```python
from build123d import *

# Parameters (mm, degrees)
SCHIZZO1_R                   = 1.5
ESTRUSIONE_ESTRUSIONE1_DEPTH = 2
TAGLIO_ESTRUSIONE1_DEPTH     = 2
ESTRUSIONE_ESTRUSIONE2_DEPTH = 2


with BuildPart() as part:
    # Schizzo1 → Estrusione-Estrusione1 (new body)
    with BuildSketch(Plane.XY):
        with BuildLine():
            Line((4.009057919, 37.078949925), (4.009057919, -12.921050075))
            ThreePointArc((4.009057919, -12.921050075), (2.544591824, -16.456583981), (-0.990942081, -17.921050075))
            Line((-0.990942081, -17.921050075), (-50.990942081, -17.921050075))
            ThreePointArc((-50.990942081, -17.921050075), (-54.526475987, -16.456583981), (-55.990942081, -12.921050075))
            Line((-55.990942081, -12.921050075), (-55.990942081, 37.078949925))
            ThreePointArc((-55.990942081, 37.078949925), (-54.526475987, 40.614483831), (-50.990942081, 42.078949925))
            Line((-50.990942081, 42.078949925), (-0.990942081, 42.078949925))
            ThreePointArc((-0.990942081, 42.078949925), (2.544591824, 40.614483831), (4.009057919, 37.078949925))
        make_face()
        with Locations((-50.990942081, 37.078949925)):
            Circle(SCHIZZO1_R, mode=Mode.SUBTRACT)
        with Locations((-0.990942081, 37.078949925)):
            Circle(SCHIZZO1_R, mode=Mode.SUBTRACT)
        with Locations((-50.990942081, -12.921050075)):
            Circle(SCHIZZO1_R, mode=Mode.SUBTRACT)
        with Locations((-0.990942081, -12.921050075)):
            Circle(SCHIZZO1_R, mode=Mode.SUBTRACT)
        with BuildLine():
            Line((-31.315733716, 32.226325066), (-29.922818488, 39.296413949))
            ThreePointArc((-29.922818488, 39.296413949), (-36.65420027, 37.427419796), (-42.697428035, 33.922560594))
            Line((-42.697428035, 33.922560594), (-36.878383255, 29.847848476))
            ThreePointArc((-36.878383255, 29.847848476), (-34.183829904, 31.240022968), (-31.315733716, 32.226325066))
        make_face(mode=Mode.SUBTRACT)
        with BuildLine():
            Line((-22.358446359, 39.337984663), (-21.125016906, 32.342042069))
            ThreePointArc((-21.125016906, 32.342042069), (-18.235263935, 31.421121146), (-15.509792769, 30.090491783))
            Line((-15.509792769, 30.090491783), (-9.525545173, 34.104859773))
            ThreePointArc((-9.525545173, 34.104859773), (-15.606929318, 37.543087038), (-22.358446359, 39.337984663))
        make_face(mode=Mode.SUBTRACT)
        with BuildLine():
            Line((-4.147331412, 28.785435879), (-8.22204353, 22.966391099))
            ThreePointArc((-8.22204353, 22.966391099), (-6.829869038, 20.271837748), (-5.84356694, 17.403741559))
            Line((-5.84356694, 17.403741559), (1.226521943, 16.010826332))
            ThreePointArc((1.226521943, 16.010826332), (-0.642472211, 22.742208114), (-4.147331412, 28.785435879))
        make_face(mode=Mode.SUBTRACT)
        with BuildLine():
            Line((1.268092656, 8.446454203), (-5.727849938, 7.213024749))
            ThreePointArc((-5.727849938, 7.213024749), (-6.648770861, 4.323271778), (-7.979400223, 1.597800612))
            Line((-7.979400223, 1.597800612), (-3.965032233, -4.386446983))
            ThreePointArc((-3.965032233, -4.386446983), (-0.526804968, 1.694937161), (1.268092656, 8.446454203))
        make_face(mode=Mode.SUBTRACT)
        with BuildLine():
            Line((-9.284456128, -9.764660744), (-15.103500908, -5.689948626))
            ThreePointArc((-15.103500908, -5.689948626), (-16.317583854, -6.379009649), (-17.575076336, -6.985239929))
            Line((-17.575076336, -6.985239929), (-22.566296054, 5.239602614))
            ThreePointArc((-22.566296054, 5.239602614), (-26.23827157, 19.723797875), (-28.966350145, 5.032545245))
            Line((-28.966350145, 5.032545245), (-34.305917557, -7.029459582))
            ThreePointArc((-34.305917557, -7.029459582), (-35.404993092, -6.512601237), (-36.472091394, -5.932591934))
            Line((-36.472091394, -5.932591934), (-42.45633899, -9.946959923))
            ThreePointArc((-42.45633899, -9.946959923), (-25.839815546, -15.420634813), (-9.284456128, -9.764660744))
        make_face(mode=Mode.SUBTRACT)
        with BuildLine():
            Line((-47.834552751, -4.627536029), (-43.759840633, 1.191508751))
            ThreePointArc((-43.759840633, 1.191508751), (-45.152015125, 3.886062102), (-46.138317223, 6.754158291))
            Line((-46.138317223, 6.754158291), (-53.208406106, 8.147073518))
            ThreePointArc((-53.208406106, 8.147073518), (-51.339411952, 1.415691736), (-47.834552751, -4.627536029))
        make_face(mode=Mode.SUBTRACT)
        with BuildLine():
            Line((-53.249976819, 15.711445647), (-46.254034225, 16.944875101))
            ThreePointArc((-46.254034225, 16.944875101), (-45.333113302, 19.834628071), (-44.00248394, 22.560099238))
            Line((-44.00248394, 22.560099238), (-48.01685193, 28.544346833))
            ThreePointArc((-48.01685193, 28.544346833), (-51.455079195, 22.462962688), (-53.249976819, 15.711445647))
        make_face(mode=Mode.SUBTRACT)
    extrude(amount=ESTRUSIONE_ESTRUSIONE1_DEPTH)

    # Schizzo2 → Taglio-Estrusione1 (cut)
    with BuildSketch(Plane.XY):
        with BuildLine():
            Line((-29.267736933, 24.477334627), (-28.432897549, 28.714770282))
            Line((-28.432897549, 28.714770282), (-23.731058754, 28.714770282))
            Line((-23.731058754, 28.714770282), (-22.996526589, 24.54854509))
            ThreePointArc((-22.996526589, 24.54854509), (-21.218217068, 23.981824522), (-19.541004043, 23.162975684))
            Line((-19.541004043, 23.162975684), (-15.954363967, 25.56897458))
            Line((-15.954363967, 25.56897458), (-12.629661871, 22.244272484))
            Line((-12.629661871, 22.244272484), (-15.056235281, 18.778913724))
            ThreePointArc((-15.056235281, 18.778913724), (-14.199512517, 17.120727047), (-13.592557379, 15.355744777))
            Line((-13.592557379, 15.355744777), (-9.355121725, 14.520905393))
            Line((-9.355121725, 14.520905393), (-9.355121725, 9.819066597))
            Line((-9.355121725, 9.819066597), (-13.521346916, 9.084534432))
            ThreePointArc((-13.521346916, 9.084534432), (-14.088067484, 7.306224912), (-14.906916322, 5.629011886))
            Line((-14.906916322, 5.629011886), (-12.500917426, 2.042371811))
            Line((-12.500917426, 2.042371811), (-15.825619522, -1.282330286))
            Line((-15.825619522, -1.282330286), (-19.290978282, 1.144243124))
            ThreePointArc((-19.290978282, 1.144243124), (-20.038106249, 0.720205572), (-20.811947777, 0.347140784))
            Line((-20.811947777, 0.347140784), (-23.883467603, 7.870120811))
            ThreePointArc((-23.883467603, 7.870120811), (-26.524135322, 16.755636376), (-27.096941459, 7.503749758))
            Line((-27.096941459, 7.503749758), (-30.402118498, 0.037403083))
            ThreePointArc((-30.402118498, 0.037403083), (-31.442562341, 0.471316046), (-32.44088012, 0.994924166))
            Line((-32.44088012, 0.994924166), (-36.027520196, -1.411074731))
            Line((-36.027520196, -1.411074731), (-39.352222292, 1.913627366))
            Line((-39.352222292, 1.913627366), (-36.925648882, 5.378986126))
            ThreePointArc((-36.925648882, 5.378986126), (-37.782371646, 7.037172803), (-38.389326784, 8.802155073))
            Line((-38.389326784, 8.802155073), (-42.626762438, 9.636994457))
            Line((-42.626762438, 9.636994457), (-42.626762438, 14.338833252))
            Line((-42.626762438, 14.338833252), (-38.460537247, 15.073365418))
            ThreePointArc((-38.460537247, 15.073365418), (-37.893816679, 16.851674938), (-37.074967841, 18.528887964))
            Line((-37.074967841, 18.528887964), (-39.480966737, 22.115528039))
            Line((-39.480966737, 22.115528039), (-36.156264641, 25.440230135))
            Line((-36.156264641, 25.440230135), (-32.690905881, 23.013656726))
            ThreePointArc((-32.690905881, 23.013656726), (-31.032719203, 23.87037949), (-29.267736933, 24.477334627))
        make_face()
    extrude(amount=TAGLIO_ESTRUSIONE1_DEPTH, mode=Mode.SUBTRACT)

    # Schizzo3 → Estrusione-Estrusione2 (add)
    with BuildSketch(Plane.XY):
        with BuildLine():
            Line((-28.179815713, 19.609421722), (-26.38592332, 28.714770282))
            Line((-26.38592332, 28.714770282), (-25.857793685, 28.714770282))
            Line((-25.857793685, 28.714770282), (-24.260309247, 19.653928262))
            ThreePointArc((-24.260309247, 19.653928262), (-23.148865797, 19.299727906), (-22.100607656, 18.787947383))
            Line((-22.100607656, 18.787947383), (-19.858957609, 20.291696693))
            Line((-19.858957609, 20.291696693), (-17.781018799, 18.213757883))
            Line((-17.781018799, 18.213757883), (-19.29762718, 16.047908658))
            ThreePointArc((-19.29762718, 16.047908658), (-18.762175452, 15.011541984), (-18.382828491, 13.908428066))
            Line((-18.382828491, 13.908428066), (-9.355121725, 12.129832289))
            Line((-9.355121725, 12.129832289), (-9.355121725, 11.572717293))
            Line((-9.355121725, 11.572717293), (-18.338321952, 9.9889216))
            ThreePointArc((-18.338321952, 9.9889216), (-18.692522307, 8.87747815), (-19.204302831, 7.829220009))
            Line((-19.204302831, 7.829220009), (-17.70055352, 5.587569962))
            Line((-17.70055352, 5.587569962), (-19.778492331, 3.509631152))
            Line((-19.778492331, 3.509631152), (-21.944341556, 5.026239533))
            ThreePointArc((-21.944341556, 5.026239533), (-22.411296535, 4.761216062), (-22.89494749, 4.52805057))
            Line((-22.89494749, 4.52805057), (-24.814647381, 9.229913087))
            ThreePointArc((-24.814647381, 9.229913087), (-26.226945656, 14.800757418), (-27.276206647, 9.150275637))
            Line((-27.276206647, 9.150275637), (-29.329886421, 4.511043011))
            ThreePointArc((-29.329886421, 4.511043011), (-29.75260778, 4.709834682), (-30.163030204, 4.932915184))
            Line((-30.163030204, 4.932915184), (-32.404680252, 3.429165873))
            Line((-32.404680252, 3.429165873), (-34.482619062, 5.507104684))
            Line((-34.482619062, 5.507104684), (-32.966010681, 7.672953909))
            ThreePointArc((-32.966010681, 7.672953909), (-33.501462408, 8.709320582), (-33.880809369, 9.812434501))
            Line((-33.880809369, 9.812434501), (-42.626762438, 11.535520506))
            Line((-42.626762438, 11.535520506), (-42.626762438, 12.197820253))
            Line((-42.626762438, 12.197820253), (-33.925315908, 13.731940966))
            ThreePointArc((-33.925315908, 13.731940966), (-33.571115553, 14.843384416), (-33.05933503, 15.891642557))
            Line((-33.05933503, 15.891642557), (-34.56308434, 18.133292605))
            Line((-34.56308434, 18.133292605), (-32.48514553, 20.211231415))
            Line((-32.48514553, 20.211231415), (-30.319296305, 18.694623034))
            ThreePointArc((-30.319296305, 18.694623034), (-29.282929631, 19.230074761), (-28.179815713, 19.609421722))
        make_face()
    extrude(amount=ESTRUSIONE_ESTRUSIONE2_DEPTH)


solid = part.part
```
The model under review builds one solid part; all positions refer to its coordinate system, in mm. Give positions to 0.01 mm unless a question says otherwise; leave off trailing zeros. Write item = value, one per line. Start each with the question number.
Q1. Mouldability with a two-part tool opening along X and no side actions: class faces 1 (the face through (-18.275, 31.437, 0.986)), 2 (the face through (-55.991, 12, 1)) as released by +X, released by -X, zero draft, split by the parting line, or undercut.
Q2. We need section A-A (z = 0.5). Give the number of separate pieces and of enclosed holes in the cut face, plus the area to 3 significant figures.
Q3. For line 1 (Y direction, x = -1.5, z = 1.05); line 2 (X direction, y = 34, z = 0.95); line 3 (Y direction, x = -42.5, z = 0.7), list the stretches that pass through material, from the lowest coordinate up.
Result set:
q1.face_1 = undercut
q1.face_2 = released by -X
q2.separate_pieces = 1
q2.enclosed_holes = 13
q2.area = 2,420 mm2
q3.line_1 = -17.92 to -14.33, -11.51 to -0.43, 7.96 to 16.55, 24.59 to 35.67, 38.49 to 42.08
q3.line_2 = -55.99 to -42.6, -30.97 to -21.42, -9.68 to 4.01
q3.line_3 = -17.92 to 9.61, 11.51 to 12.22, 14.36 to 33.78, 34.07 to 42.08
